Autodesk Inventor part; units mm, degrees
ref_plane "YZ Plane" through (0, 0, 0) normal (1, 0, 0) x (0, 1, 0)
ref_plane "XZ Plane" through (0, 0, 0) normal (0, 1, 0) x (-1, 0, 0)
ref_plane "XY Plane" through (0, 0, 0) normal (0, 0, 1) x (1, 0, 0)
sketch "Sketch1" plane through (0, 0, 0) normal (0, 1, 0) x (-1, 0, 0)
  line L0 (-15, 5) -> (15, 5)
  line L1 (15, 5) -> (15, -5)
  line L2 (15, -5) -> (-15, -5)
  line L3 (-15, -5) -> (-15, 5)
  line L4 (-15, 5) -> (15, -5) construction
  line L5 (15, 5) -> (-15, -5) construction
  point P0 (0, 0)
  dimension "d0" = 30
  dimension "d1" = 10
extrude "Extrusion1" add sketch "Sketch1" along normal blind 30
sketch "Sketch2" plane through (15, 0, -5) normal (0, 0, -1) x (-1, 0, 0)
  line L0 (0, 0) -> (0, 30)
  line L1 (0, 30) -> (30, 30)
  line L2 (0, 0) -> (30, 30)
  line L3 (10, 5) -> (20, 5)
  line L4 (20, 5) -> (20, 25)
  line L5 (20, 25) -> (10, 25)
  line L6 (10, 25) -> (10, 5)
  line L7 (10, 5) -> (20, 25) construction
  line L8 (20, 5) -> (10, 25) construction
  point P0 (15, 0)
  point P1 (15, 15)
  dimension "d4" = 10
  dimension "d5" = 20
extrude "Extrusion2" cut sketch "Sketch2" against normal through all contours L6 L5 L4 L2 | L2 L4 L3 L6
sketch "Sketch3" plane through (15, 0, 5) normal (1, 0, 0) x (0, 0, -1)
  line L0 (10, 0) -> (0, 0)
  line L1 (0, 30) -> (10, 30)
  line L2 (0, 0) -> (10, 30)
  line L3 (5, 15) -> (17.6725, 15)
  point P0 (5, 0)
hole "Hole1" at (15, 15, 0) direction (-1, 0, 0) diameter 3.4 depth 10 countersink diameter 5.9 countersink angle 90
sketch "Sketch4" plane through (-5, 5, -5) normal (1, 0, 0) x (0, 0, -1)
  line L0 (-10, 0) -> (-10, 20)
  line L1 (0, 20) -> (-10, 20)
  line L2 (-10, 0) -> (0, 20)
  line L3 (-5, 10) -> (5, 10)
  point P0 (-5, -5)
  dimension "d15" = 10
hole "Hole2" at (-5, 15, 0) direction (-1, 0, 0) diameter 3.4 depth 9 counterbore diameter 4.1 counterbore depth 5.1
sketch "Sketch5" plane through (15, 0, -5) normal (0, 0, -1) x (-1, 0, 0)
  line L0 (30, 0) -> (0, 0)
  line L1 (30, 0) -> (30, 30)
  line L2 (0, 0) -> (30, 30)
  line L3 (5, 10) -> (25, 10)
  line L4 (25, 10) -> (25, 20)
  line L5 (25, 20) -> (5, 20)
  line L6 (5, 20) -> (5, 10)
  line L7 (5, 10) -> (25, 20) construction
  line L8 (25, 10) -> (5, 20) construction
  point P0 (15, 0)
  point P1 (15, 15)
  dimension "d23" = 20
  dimension "d24" = 10
hole "Hole3" at (10, 20, -5) at (10, 10, -5) at (-10, 10, -5) at (-10, 20, -5) direction (0, 0, 1) diameter 3.4 end through all countersink diameter 5.9 countersink angle 90
fillet "Fillet1" radius 6 6 edges at (15, 30, 0) (-15, 30, 0) (15, 0, 0) (-15, 0, 0) (0, 30, -5) (0, 0, -5)
fillet "Fillet2" radius 2 6 edges at (13.2426, 28.2426, -3.2426) (13.2426, 1.7574, -3.2426) (15, 15, -5) (-13.2426, 28.2426, -3.2426) (-13.2426, 1.7574, -3.2426) (-15, 15, -5)
properties part number "Tensor"
Geometry check sheet. Reference: the model listing, model coordinates, mm. A direction names the side the tool comes from. Round coordinates to 2 decimals unless told otherwise and drop trailing zeros. Loops run counter-clockwise (first coordinate to the right, second up) from the corner with the lowest first, then second, coordinate; pieces in that order, holes last.
Item 1: Access from +Z, -Z, +X, -X, +Y, -Y to the whole of each face (thin tool, end or side, straight path). Record for faces 5 (the flat face through (0, 5, 0)), 6 (the flat face through (-8, 15, -5)).
Item 2: Thickness scan on line 1 (X direction, y = 10, z = 2); line 2 (Z direction, x = 8.25, y = 15); line 3 (X direction, y = 18.5, z = -2.5). Record the ranges inside material, lowest first.
Item 3: Cross-section at C-C on x = 6. Record the boundary of the cut face in (y, z).
Item 4: Cross-section at D-D on z = 3.5. Record the boundary of the cut face in (x, y).
Item 5: Gauge pin test, flat ends, axial feed: pin 1 (5 mm diameter, centred on x = -1, z = -4, fed in from -Y); pin 2 (4.5 mm diameter, centred on x = -10, y = 10, fed in from -Z); pin 3 (4 mm diameter, centred on y = 15, z = 0, fed in from +X). Record the tip position at first contact, or that the pin passes through.
Item 6: Cross-section at B-B on y = 15. Record the boundary of the cut face in (x, z).
Item 7: Cross-section at A-A on y = 10. Record the boundary of the cut face in (x, z).
Item 8: Mould release check, pull along Z, two halves, no side actions. Record for faces 1 (the cylindrical face through (10.65, 21.57, 0.69)), 2 (the cylindrical face through (9.314, 13.314, 0.221)), 3 (the cylindrical face through (-12.077, 13.314, 0.221)), 4 (the cylindrical face through (-0.182, 28.289, -3.196)): pulls with the +Z half, pulls with the -Z half, needs draft (parallel to the pull), parting line crosses it, or undercut.
Answer sheet:
1. face 5: +Z, -Z
1. face 6: -Z, +X, -X, +Y, -Y
2. line 1: x = -15 to -11.7, -8.3 to -5, 5 to 8.3, 11.7 to 15
2. line 2: z = -5 to -1.7, 1.7 to 5
2. line 3: x = -15 to -10.8, -9.2 to -5, 5 to 9.2, 10.8 to 15
3. outline: (0, 1) arc R6 ccw to (6, -5) - (24, -5) arc R6 ccw to (30, 1) - (30, 5) - (0, 5) - close; hole circle Ø3.4 at (15, 0)
4. outline: (-15, 6) arc R6 ccw to (-9, 0) - (9, 0) arc R6 ccw to (15, 6) - (15, 24) arc R6 ccw to (9, 30) - (-9, 30) arc R6 ccw to (-15, 24) - close; hole circle Ø3.4 at (-10, 10); hole circle Ø3.4 at (-10, 20); hole (-5, 5) - (5, 5) - (5, 25) - (-5, 25) - close; hole circle Ø3.4 at (10, 10); hole circle Ø3.4 at (10, 20)
5. pin 1: stops at y = 0.55
5. pin 2: stops at z = -4.3
5. pin 3: stops at x = 14.05
6. outline: (-15, -3) arc R2 ccw to (-13, -5) - (-5, -5) - (-5, -2.05) - (-10.1, -2.05) - (-10.1, -1.7) - (-14, -1.7) - (-14, 1.7) - (-10.1, 1.7) - (-10.1, 2.05) - (-5, 2.05) - (-5, 5) - (-15, 5) - close; (5, -5) - (13, -5) arc R2 ccw to (15, -3) - (15, -2.95) - (13.75, -1.7) - (5, -1.7) - close; (5, 1.7) - (13.75, 1.7) - (15, 2.95) - (15, 5) - (5, 5) - close
7. outline: (-15, -3) arc R2 ccw to (-13, -5) - (-12.95, -5) - (-11.7, -3.75) - (-11.7, 5) - (-15, 5) - close; (-8.3, -3.75) - (-7.05, -5) - (-5, -5) - (-5, 5) - (-8.3, 5) - close; (5, -5) - (7.05, -5) - (8.3, -3.75) - (8.3, 5) - (5, 5) - close; (11.7, -3.75) - (12.95, -5) - (13, -5) arc R2 ccw to (15, -3) - (15, 5) - (11.7, 5) - close
8. face 1: needs draft
8. face 2: undercut
8. face 3: undercut
8. face 4: pulls with the -Z half
